Source: CAD feature listing. Evaluate the final solid. Frame: model axes, mm. Face numbers are marked on the shaded views. A direction names the side the tool comes from. Coordinates: 2 decimals unless noted, no trailing zeros. Order: outer loops, then holes, each group sorted by start corner. A loop starts at its lowest first (then second) coordinate and runs counter-clockwise, first axis right, second up. Notation, with made-up numbers: (9, 23) -> (17, 23) arc R17 ccw to (17, 53) -> close; hole circle Ø9 at (-14, 69). An arc over 180 degrees is marked (long way). Write each question's results on one line, items separated by ' | '. Start each with the question number.
from build123d import *

# Parameters (mm, degrees)
BOSS_EXTRUDE1_DEPTH = 6.35
BOSS_EXTRUDE2_DEPTH = 12.7
SKETCH5_R           = 6.35
CUT_EXTRUDE2_DEPTH  = 13.7


with BuildPart() as part:
    # Sketch2 → Boss-Extrude1 (new body, symmetric)
    with BuildSketch(Plane(origin=(0, 0, 0), x_dir=(0, 0, -1), z_dir=(1, 0, 0))):
        Polygon((0, 31.75), (0, 0), (31.3944, 0), (31.3944, -2.9972), (74.9808, -2.9972), (61.24296189, 34.7472), (31.3944, 34.7472), (31.3944, 31.75), align=None)
    extrude(amount=BOSS_EXTRUDE1_DEPTH, both=True)

    # Sketch4 → Boss-Extrude2 (add, through all)
    with BuildSketch(Plane(origin=(6.35, 0, 0), x_dir=(0, 0, -1), z_dir=(1, 0, 0))):
        with BuildLine():
            Line((57.141767732, 34.7472), (61.24296189, 34.7472))
            Line((61.24296189, 34.7472), (57.249189303, 45.72))
            Line((57.249189303, 45.72), (38.914198342, 45.72))
            ThreePointArc((38.914198342, 45.72), (34.700855885, 42.429053325), (32.215182454, 37.695765645))
            Line((32.215182454, 37.695765645), (31.3944, 34.7472))
            Line((31.3944, 34.7472), (31.758232268, 34.7472))
            ThreePointArc((31.758232268, 34.7472), (44.45, 21.59), (57.141767732, 34.7472))
        make_face()
    extrude(amount=-BOSS_EXTRUDE2_DEPTH)

    # Sketch5 → Cut-Extrude2 (cut, through all)
    with BuildSketch(Plane(origin=(6.35, 0, 0), x_dir=(0, 0, -1), z_dir=(1, 0, 0))):
        with Locations((44.45, 34.29)):
            Circle(SKETCH5_R)
    extrude(amount=-CUT_EXTRUDE2_DEPTH, mode=Mode.SUBTRACT)


solid = part.part
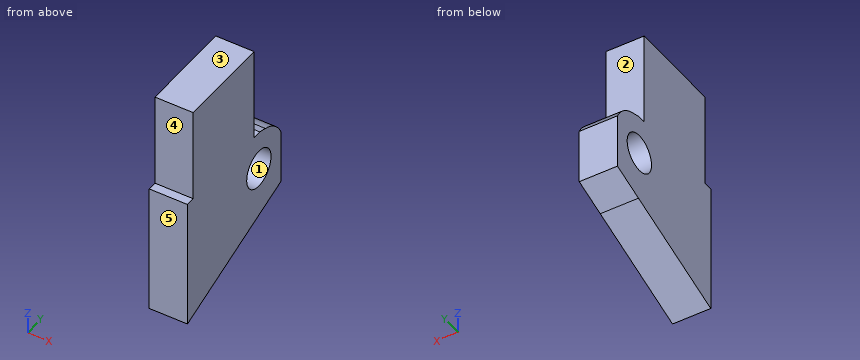
(1) Section C-C on y = 24.5. Return the cut outline in (x, z), then the cut area to 3 significant figures.
(2) Reachability of the marked faces 4 and 5 from +Z, -Z, +X, -X, +Y, -Y: full face, straight path, thin tool, end or side. Return the list, or none.
(3) Section D-D on z = -22.5. Return the cut outline in (x, y).
(4) Line query: L1, parallel to Y at x = -2.5, z = -44.45; L2, parallel to Y at x = 3.75, z = -42; L3, parallel to Z at x = -1, y = 36. Output: solid intervals per line, ascending.
(5) Section B-B on x = -2.75. Return the cut outline in (y, z).
(6) Section A-A on z = -44.45. Return the cut outline in (x, y), then the cut area to 3 significant figures.
(7) Draft query along Z for the marked faces 1, 2 and 3. Return one class per face: released by +Z, released by -Z, zero draft, split by the parting line, or undercut.
(8) First-contact query: P1, Ø0.9, axis at x = 1, y = 34, coming from the +Z side; P2, Ø2, axis at x = 3, y = 11, coming from the -Z side; P3, Ø4, axis at x = 2, y = 13, coming from the -Z side. Flat tips, straight axial feed; report the tip coordinate or a pass-through.
Results list:
1) outline: (-6.35, -64.97) -> (6.35, -64.97) -> (6.35, 0) -> (-6.35, 0) -> close | area: 825 mm²
2) face 4: +Z, +X, -X, -Y | face 5: +Z, -Z, +X, -X, -Y
3) outline: (-6.35, 0) -> (6.35, 0) -> (6.35, 31.75) -> (-6.35, 31.75) -> close
4) L1: y = -3 to 27.94, 40.64 to 45.72 | L2: y = -3 to 28.43, 40.15 to 45.72 | L3: z = -60.79 to -50.57, -38.33 to -31.74
5) outline: (-3, -74.98) -> (45.72, -57.25) -> (45.72, -38.91) arc R12.7 ccw to (37.7, -32.22) -> (34.75, -31.39) -> (31.75, -31.39) -> (31.75, 0) -> (0, 0) -> (0, -31.39) -> (-3, -31.39) -> close; hole circle Ø12.7 at (34.29, -44.45)
6) outline: (-6.35, -3) -> (6.35, -3) -> (6.35, 27.94) -> (-6.35, 27.94) -> close; (-6.35, 40.64) -> (6.35, 40.64) -> (6.35, 45.72) -> (-6.35, 45.72) -> close | area: 457 mm²
7) face 1: undercut | face 2: zero draft | face 3: released by +Z
8) P1: stops at z = -31.39 | P2: stops at z = -70.25 | P3: stops at z = -69.89
